Answer from the drawing. Dimensions are ordinates in mm from the lowest x, y and z of the part. Round coordinates to 2 decimals unless told otherwise and drop trailing zeros. Order: outer loops, then holes, each group sorted by start corner. A loop starts at its lowest first (then second) coordinate and runs counter-clockwise, first axis right, second up. Notation, with made-up numbers: (-15, -34.75) -> (42, -34.75) arc R11 ccw to (42, -14.75) -> close; hole circle Ø6 at (-24, 26.5). An arc over 180 degrees is marked (long way). Use a Markdown table: item, result. Add a question column.
Item 1: A cutting plane is placed at B-B, the plane z = 4. Give the number of separate pieces and of enclosed holes in the cut face, plus the area to 3 significant figures.
Item 2: A cutting plane is placed at C-C, the plane y = 108.5. Determine the outline of the cut face in (x, z).
Item 3: Find the intervals of material crossed by L1, parallel to X at y = 81.92, z = 2 (1 decimal); L2, parallel to Y at x = 44.5, z = 2; L3, parallel to X at y = 108.5, z = 2.25, in increasing order. Write a range as [from, to].
Item 4: A cutting plane is placed at A-A, the plane x = 38.1. Determine the outline of the cut face in (y, z), plus the area to 3 significant figures.
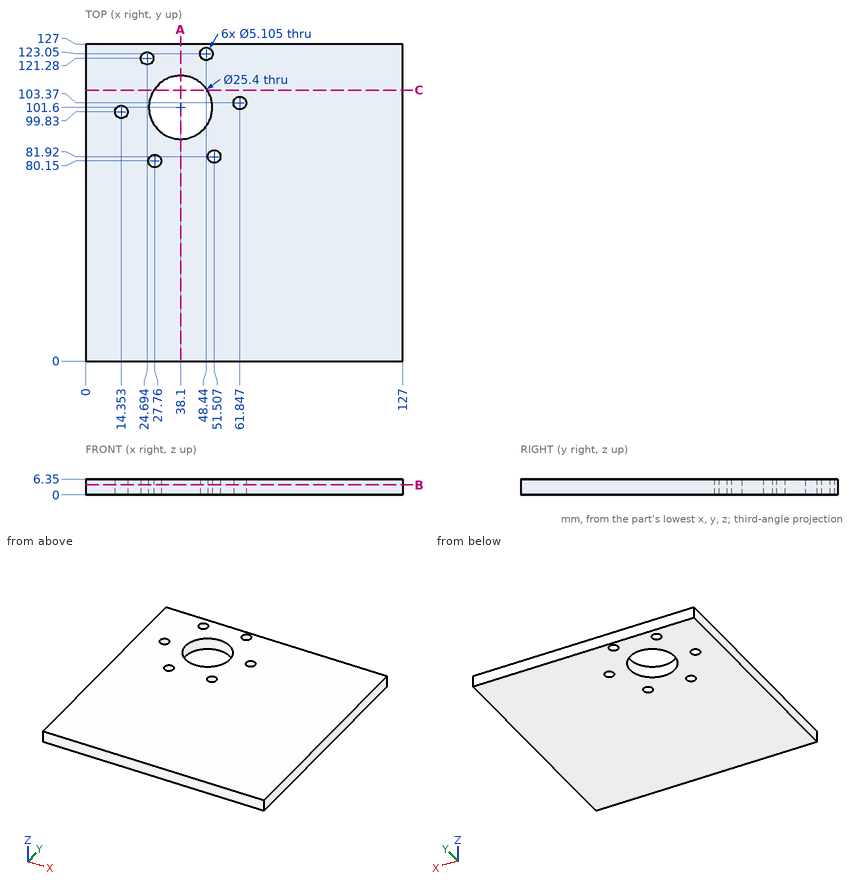
Reported:
| question | item | result |
|---|---|---|
| 1 | separate pieces | 1 |
| 1 | enclosed holes | 7 |
| 1 | area | 15,500 mm² |
| 2 | outline | (0, 0) -> (27.44, 0) -> (27.44, 6.35) -> (0, 6.35) -> close; (48.76, 0) -> (127, 0) -> (127, 6.35) -> (48.76, 6.35) -> close |
| 3 | L1 | [0, 25.9], [29.6, 49], [54.1, 127] |
| 3 | L2 | [0, 90.63], [112.57, 127] |
| 3 | L3 | [0, 27.44], [48.76, 127] |
| 4 | outline | (0, 0) -> (88.9, 0) -> (88.9, 6.35) -> (0, 6.35) -> close; (114.3, 0) -> (127, 0) -> (127, 6.35) -> (114.3, 6.35) -> close |
| 4 | area | 645 mm² |
